Can you work these out from the model? Positions are in its coordinate system, mm. Face numbers are marked on the shaded views. A direction names the side the tool comes from. Round coordinates to 2 decimals unless told otherwise and drop trailing zeros. Loops run counter-clockwise (first coordinate to the right, second up) from the corner with the lowest first, then second, coordinate; pieces in that order, holes last.
from build123d import *

# Parameters (mm, degrees)
SKETCH1_W                      = 18.669
SKETCH1_H                      = 44.069
BOSS_EXTRUDE1_DEPTH            = 12.7
TAP_DRILL_FOR_10_32_TAP1_D     = 4.0386
TAP_DRILL_FOR_10_32_TAP2_D     = 4.0386
TAP_DRILL_FOR_10_32_TAP2_DEPTH = 6.35
TAP_DRILL_FOR_10_32_TAP2_TIP   = 1.213317848


with BuildPart() as part:
    # Sketch1 → Boss-Extrude1 (new body)
    with BuildSketch(Plane.XY):
        Rectangle(SKETCH1_W, SKETCH1_H)
    extrude(amount=BOSS_EXTRUDE1_DEPTH)

    # Tap Drill for #10-32 Tap1 (through all)
    with Locations(Plane(origin=(9.3345, 0, 0), x_dir=(0, 0, -1), z_dir=(1, 0, 0))):
        with Locations((-6.35, 8.89), (-6.35, -8.89)):
            Hole(TAP_DRILL_FOR_10_32_TAP1_D / 2)

    # Tap Drill for #10-32 Tap2
    with Locations(Plane.XY.offset(12.7)):
        with Locations((0, 16.51), (0, -16.51)):
            Hole(TAP_DRILL_FOR_10_32_TAP2_D / 2, depth=TAP_DRILL_FOR_10_32_TAP2_DEPTH)
            with Locations((0, 0, -(TAP_DRILL_FOR_10_32_TAP2_DEPTH + TAP_DRILL_FOR_10_32_TAP2_TIP / 2))):  # 118° drill point
                Cone(0, TAP_DRILL_FOR_10_32_TAP2_D / 2, TAP_DRILL_FOR_10_32_TAP2_TIP, mode=Mode.SUBTRACT)


solid = part.part
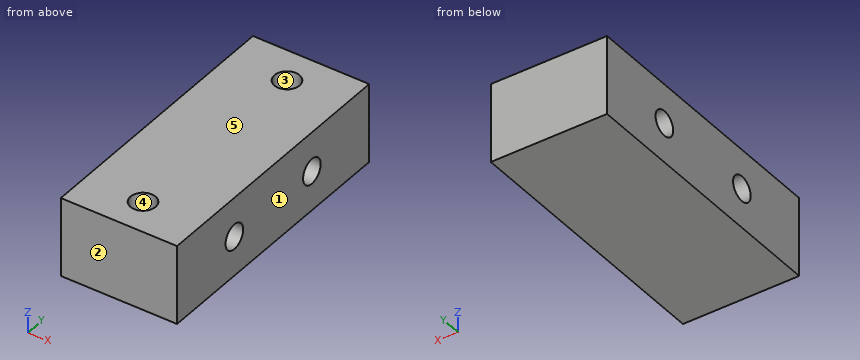
(1) Will these pins go through, and if not, where does the flat tip stop? P1, Ø2, axis at x = 3.5, y = 10, coming from the -Z side; P2, Ø3.5, axis at x = 0, y = 16.51, coming from the +Z side.
Worked answers:
P1: stops at z = 0
P2: stops at z = 6.19
(2) If we section it at D-D, the plane z = 11.75: List the corners of the cut face in (x, y) for me, then the cut area to 3 significant figures.
Worked answers:
outline: (-9.33, -22.03) - (9.33, -22.03) - (9.33, 22.03) - (-9.33, 22.03) - close; hole circle Ø4.04 at (0, -16.51); hole circle Ø4.04 at (0, 16.51)
area: 797 mm2
(3) If I drill on line 1 (Y direction, x = 0, z = 9.75); line 2 (Y direction, x = -4.5, z = 6.35); line 3 (X direction, y = -16.51, z = 11.25), over which ranges is the centre line in solid material (lowest first)?
Worked answers:
line 1: y = -22.03 to -18.53, -14.49 to 14.49, 18.53 to 22.03
line 2: y = -22.03 to -10.91, -6.87 to 6.87, 10.91 to 22.03
line 3: x = -9.33 to -2.02, 2.02 to 9.33
(4) If we mould it in two halves opening along X, with no side actions, what happens to the marked faces 1, 2 and 3? For each: released by +X, released by -X, zero draft, split by the parting line, or undercut.
Worked answers:
face 1: released by +X
face 2: zero draft
face 3: undercut
(5) If we section it at C-C, the plane x = 3.5: List the corners of the cut face in (y, z) for me.
Worked answers:
outline: (-22.03, 0) - (22.03, 0) - (22.03, 12.7) - (-22.03, 12.7) - close; hole circle Ø4.04 at (-8.89, 6.35); hole circle Ø4.04 at (8.89, 6.35)
(6) If we section it at A-A, the plane y = -8.89: List the corners of the cut face in (x, z) for me.
Worked answers:
outline: (-9.33, 0) - (9.33, 0) - (9.33, 4.33) - (-9.33, 4.33) - close; (-9.33, 8.37) - (9.33, 8.37) - (9.33, 12.7) - (-9.33, 12.7) - close
(7) If we section it at B-B, the plane z = 7: List the corners of the cut face in (x, y) for me.
Worked answers:
outline: (-9.33, -22.03) - (9.33, -22.03) - (9.33, -10.8) - (-9.33, -10.8) - close; (-9.33, -6.98) - (9.33, -6.98) - (9.33, 6.98) - (-9.33, 6.98) - close; (-9.33, 10.8) - (9.33, 10.8) - (9.33, 22.03) - (-9.33, 22.03) - close; hole circle Ø4.04 at (0, -16.51); hole circle Ø4.04 at (0, 16.51)
(8) For the marked faces 4 and 5, which set-ups out of +Z, -Z, +X, -X, +Y, -Y let a thin tool reach every point of the face, with its end or its side?
Worked answers:
face 4: +Z
face 5: +Z, +X, -X, +Y, -Y
